Part print with two shaded views. Sizes in mm from the minimum x, y, z corner. Give positions to 0.01 mm unless a question says otherwise; leave off trailing zeros. Loops run counter-clockwise (first coordinate to the right, second up) from the corner with the lowest first, then second, coordinate; pieces in that order, holes last. Notation, with made-up numbers: M -36,-16.5 L -16,-16.5 A26 ccw -16,-0.5 Z; hole C 35.5,59 d11. An arc over 180 degrees is marked long. Answer in a Markdown table with one row per item.
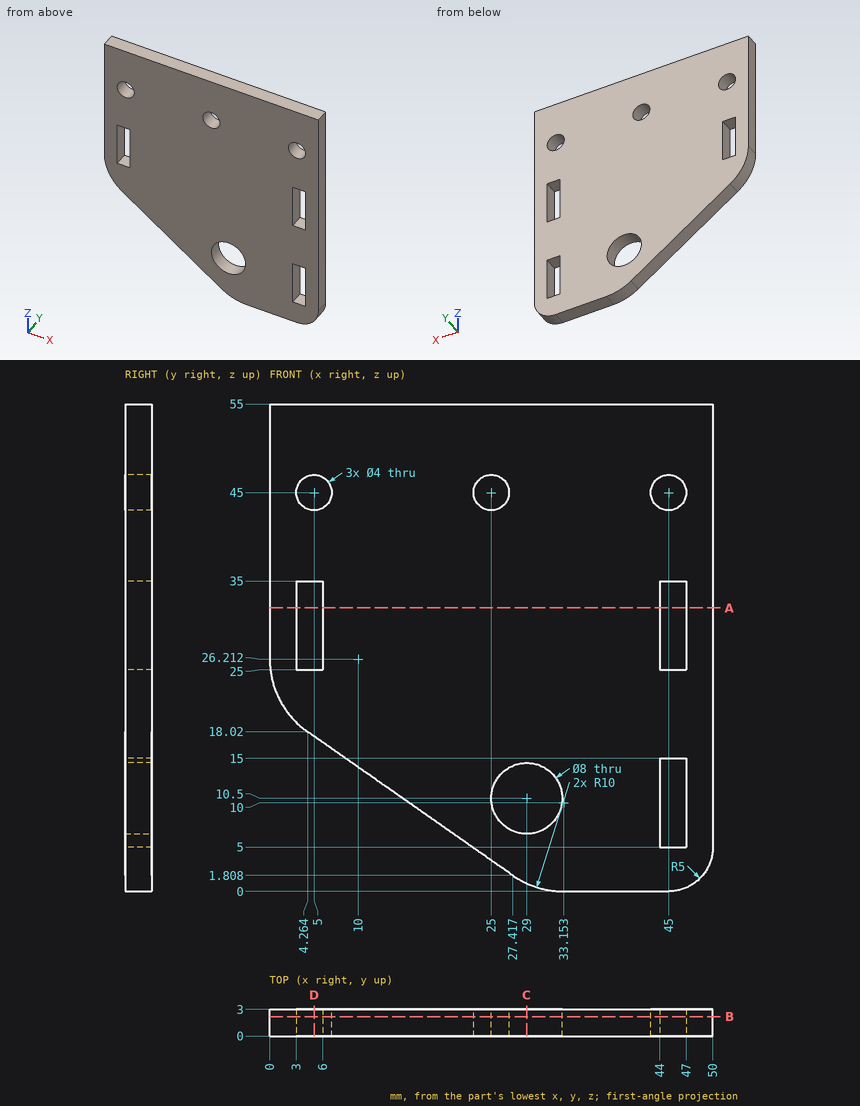
Q1. Saw through at B-B (y = 2.2). Give the cut face in (x, z) (1 decimal), and give its area (3 significant figures).
Reported:
| item | result |
|---|---|
| outline | M 0,26.2 A10 ccw 4.3,18 L 27.4,1.8 A10 ccw 33.2,0 L 45,0 A5 ccw 50,5 L 50,55 L 0,55 Z; hole M 3,25 L 6,25 L 6,35 L 3,35 Z; hole C 5,45 d4; hole C 25,45 d4; hole C 29,10.5 d8; hole C 45,45 d4; hole M 44,5 L 47,5 L 47,15 L 44,15 Z; hole M 44,25 L 47,25 L 47,35 L 44,35 Z |
| area | 2,250 mm² |
Q2. Saw through at D-D (x = 5). Give the cut face in (y, z) (1 decimal).
Reported:
| item | result |
|---|---|
| outline | M 0,17.5 L 3,17.5 L 3,25 L 0,25 Z; M 0,35 L 3,35 L 3,43 L 0,43 Z; M 0,47 L 3,47 L 3,55 L 0,55 Z |
Q3. Saw through at A-A (z = 32). Give the cut face in (x, y), and give its area (3 significant figures).
Reported:
| item | result |
|---|---|
| outline | M 0,0 L 3,0 L 3,3 L 0,3 Z; M 6,0 L 44,0 L 44,3 L 6,3 Z; M 47,0 L 50,0 L 50,3 L 47,3 Z |
| area | 132 mm² |
Q4. Probe probe 1 along X at (y, z) = (2.45, 34); probe 2 along X at (y, z) = (2, 10.5) (1 decimal); probe 3 along X at (y, z) = (2.1, 45). List the from-to ranges inside material, lowest first.
Reported:
| item | result |
|---|---|
| probe 1 | 0 to 3, 6 to 44, 47 to 50 |
| probe 2 | 15 to 25, 33 to 44, 47 to 50 |
| probe 3 | 0 to 3, 7 to 23, 27 to 43, 47 to 50 |
Q5. Saw through at C-C (x = 29). Give the cut face in (y, z), and give its area (3 significant figures).
Reported:
| item | result |
|---|---|
| outline | M 0,0.9 L 3,0.9 L 3,6.5 L 0,6.5 Z; M 0,14.5 L 3,14.5 L 3,55 L 0,55 Z |
| area | 138 mm² |
